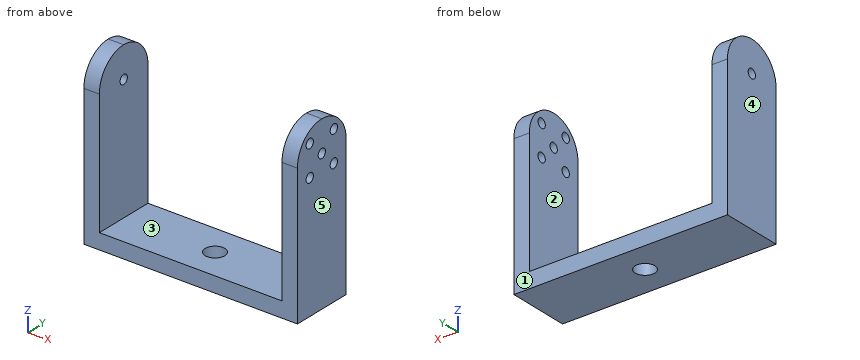
from build123d import *

# Parameters (mm, degrees)
SKETCH_1_W          = 69
SKETCH_1_H          = 20
EXTRUDE_1_DEPTH     = 5
SKETCH_2_W          = 5
SKETCH_2_H          = 20
EXTRUDE_2_DEPTH     = 50
FILLET_1_R          = 10
SKETCH_3_R          = 1.5
CUT_EXTRUDE_1_DEPTH = 82
SKETCH_4_R          = 1.5
CUT_EXTRUDE_2_DEPTH = 10
SKETCH_5_R          = 3.175
CUT_EXTRUDE_3_DEPTH = 10


with BuildPart() as part:
    # 草图1 → 凸台-拉伸1 (new body)
    with BuildSketch(Plane.XY):
        Rectangle(SKETCH_1_W, SKETCH_1_H)
    extrude(amount=EXTRUDE_1_DEPTH)

    # 草图2 → 凸台-拉伸2 (add)
    with BuildSketch(Plane.XY.offset(5)):
        with Locations((-32, 0)):
            Rectangle(SKETCH_2_W, SKETCH_2_H)
        with Locations((32, 0)):
            Rectangle(SKETCH_2_W, SKETCH_2_H)
    extrude(amount=EXTRUDE_2_DEPTH)

    # 圆角1
    fillet_1_edges = [part.edges().sort_by_distance(p)[0] for p in [
        (-32, -10, 55),
        (-32, 10, 55),
        (32, 10, 55),
        (32, -10, 55),
    ]]
    fillet(fillet_1_edges, radius=FILLET_1_R - 0.0001)  # a hair under: the kernel refuses the full size

    # 草图3 → 切除-拉伸1 (cut)
    with BuildSketch(Plane(origin=(34.5, 0, 0), x_dir=(0, 0, -1), z_dir=(1, 0, 0))):
        with Locations((-45, 0)):
            Circle(SKETCH_3_R)
    extrude(amount=-CUT_EXTRUDE_1_DEPTH, mode=Mode.SUBTRACT)

    # 草图4 → 切除-拉伸2 (cut)
    with BuildSketch(Plane(origin=(34.5, 0, 0), x_dir=(0, 0, -1), z_dir=(1, 0, 0))):
        with Locations((-49.949747468, 4.949747468)):
            Circle(SKETCH_4_R)
        with Locations((-40.050252532, 4.949747468)):
            Circle(SKETCH_4_R)
        with Locations((-40.050252532, -4.949747468)):
            Circle(SKETCH_4_R)
        with Locations((-49.949747468, -4.949747468)):
            Circle(SKETCH_4_R)
    extrude(amount=-CUT_EXTRUDE_2_DEPTH, mode=Mode.SUBTRACT)

    # 草图5 → 切除-拉伸3 (cut)
    with BuildSketch(Plane(origin=(0, 0, 0), x_dir=(-1, 0, 0), z_dir=(0, 0, -1))):
        Circle(SKETCH_5_R)
    extrude(amount=-CUT_EXTRUDE_3_DEPTH, mode=Mode.SUBTRACT)


solid = part.part
For this review, take the finished solid that the model builds, in its own axes (mm). Face numbers are marked on the shaded views. A direction names the side the tool comes from. Round coordinates to 2 decimals unless told otherwise and drop trailing zeros. Loops run counter-clockwise (first coordinate to the right, second up) from the corner with the lowest first, then second, coordinate; pieces in that order, holes last. Notation, with made-up numbers: (55.5, 43) - (84.5, 43) arc R33 ccw to (84.5, 77) - close; hole circle Ø11 at (-23, 66). An arc over 180 degrees is marked (long way). One line per question, with ' | ' between items.
Q1. Take a section at D-D (x = -20.5). Give the boundary of the cut face in (y, z), and give its area (3 significant figures).
Taken from the geometry:
outline: (-10, 0) - (10, 0) - (10, 5) - (-10, 5) - close | area: 100 mm²
Q2. For line 1 along X through (y, z) = (3.75, 11.5); line 2 along Y through (x, z) = (-33, 45); line 3 along Y through (x, z) = (0, 1) (3 decimals), list the stretches that pass through material, from the lowest coordinate up. Write a range as [from, to].
Taken from the geometry:
line 1: x = [-34.5, -29.5], [29.5, 34.5] | line 2: y = [-10, -1.5], [1.5, 10] | line 3: y = [-10, -3.175], [3.175, 10]
Q3. Take a section at B-B (x = 0). Give the boundary of the cut face in (y, z) (3 decimals), and give its area (4 significant figures).
Taken from the geometry:
outline: (-10, 0) - (-3.175, 0) - (-3.175, 5) - (-10, 5) - close; (3.175, 0) - (10, 0) - (10, 5) - (3.175, 5) - close | area: 68.25 mm²
Q4. Take a section at A-A (z = 6). Give the boundary of the cut face in (x, y), and give its area (3 significant figures).
Taken from the geometry:
outline: (-34.5, -10) - (-29.5, -10) - (-29.5, 10) - (-34.5, 10) - close; (29.5, -10) - (34.5, -10) - (34.5, 10) - (29.5, 10) - close | area: 200 mm²
Q5. Take a section at C-C (y = 8.5). Give the boundary of the cut face in (x, z).
Taken from the geometry:
outline: (-34.5, 0) - (34.5, 0) - (34.5, 50.27) - (29.5, 50.27) - (29.5, 5) - (-29.5, 5) - (-29.5, 50.27) - (-34.5, 50.27) - close
Q6. The part is to be moulded in two halves that separate along X. For the marked faces 3, 4 and 5, say which applies: released by +X, released by -X, zero draft, split by the parting line, or undercut.
Taken from the geometry:
face 3: undercut | face 4: released by -X | face 5: released by +X
Q7. Tool access review of the marked faces 1 and 2: name each direction out of +Z, -Z, +X, -X, +Y, -Y from which nothing blocks a thin tool from reaching the whole face with its end or side.
Taken from the geometry:
face 1: +Z, -Z, +X, -X, +Y | face 2: +Z, +Y, -Y
Q8. For pin 1 (10 mm diameter, centred on x = 11.5, y = 4, fed in from +Z); pin 2 (2 mm diameter, centred on x = 12, y = -0.5, fed in from -Z); pin 3 (2.5 mm diameter, centred on y = -4.95, z = 40.05, fed in from +X), all flat-tipped, find the tip position at first contact; note any pin that passes through.
Taken from the geometry:
pin 1: stops at z = 5 | pin 2: stops at z = 0 | pin 3: stops at x = -29.5
